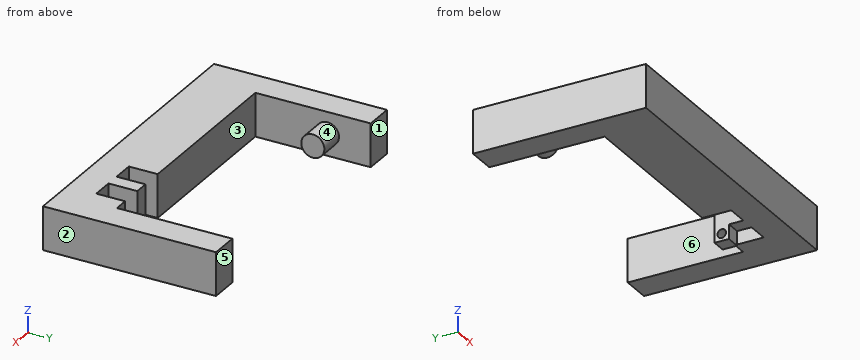
```python
from build123d import *

# Parameters (mm, degrees)
SKETCH1_3_W           = 7.5
SKETCH1_3_H           = 15
BOSS_EXTRUDE2_DEPTH   = 10
BOSS_EXTRUDE2_2_DEPTH = 10
SKETCH1_W             = 5
SKETCH1_H             = 15
SKETCH1_W_2           = 60
BOSS_EXTRUDE3_DEPTH   = 20
SKETCH2_W             = 5
SKETCH2_H             = 5
BOSS_EXTRUDE5_DEPTH   = 5
SKETCH1_9_W           = 10
SKETCH1_9_H           = 15
BOSS_EXTRUDE6_DEPTH   = 60
SKETCH4_R             = 4
BOSS_EXTRUDE7_DEPTH   = 9
SKETCH5_R             = 1.5
CUT_EXTRUDE1_DEPTH    = 5


with BuildPart() as part:
    # Sketch1<3> → Boss-Extrude2 (new body)
    with BuildSketch(Plane(origin=(0, 0, 0), x_dir=(1, 0, 0), z_dir=(0, 1, 0))):
        with Locations((36.25, 0)):
            Rectangle(SKETCH1_3_W, SKETCH1_3_H)
    extrude(amount=BOSS_EXTRUDE2_DEPTH)



with BuildPart() as body_2:
    # Sketch1<3> → Boss-Extrude2 2 (new body)
    with BuildSketch(Plane(origin=(0, 0, 0), x_dir=(1, 0, 0), z_dir=(0, 1, 0))):
        with Locations((23.75, 0)):
            Rectangle(SKETCH1_3_W, SKETCH1_3_H)
    extrude(amount=BOSS_EXTRUDE2_2_DEPTH)


with BuildPart() as part_1:
    add(part.part)

    add(body_2.part)  # Boss-Extrude3 merges body 2
    # Sketch1 → Boss-Extrude3 (add)
    with BuildSketch(Plane(origin=(0, 0, 0), x_dir=(1, 0, 0), z_dir=(0, 1, 0))):
        with Locations((30, 0)):
            Rectangle(SKETCH1_W, SKETCH1_H)
        with Locations((-10, 0)):
            Rectangle(SKETCH1_W_2, SKETCH1_H)
        with Locations((42.5, 0)):
            Rectangle(SKETCH1_W, SKETCH1_H)
    extrude(amount=BOSS_EXTRUDE3_DEPTH)

    # Sketch2 → Boss-Extrude5 (add)
    with BuildSketch(Plane(origin=(0, 0, -7.5), x_dir=(-1, 0, 0), z_dir=(0, 0, -1))):
        with Locations((-30, 17.5)):
            Rectangle(SKETCH2_W, SKETCH2_H)
    extrude(amount=BOSS_EXTRUDE5_DEPTH)

    # Sketch1<9> → Boss-Extrude6 (add)
    with BuildSketch(Plane(origin=(0, 0, 0), x_dir=(1, 0, 0), z_dir=(0, 1, 0))):
        with Locations((50, 0)):
            Rectangle(SKETCH1_9_W, SKETCH1_9_H)
        with Locations((-45, 0)):
            Rectangle(SKETCH1_9_W, SKETCH1_9_H)
    extrude(amount=BOSS_EXTRUDE6_DEPTH)

    # Sketch4 → Boss-Extrude7 (add)
    with BuildSketch(Plane(origin=(-40, 0, 0), x_dir=(0, 0, -1), z_dir=(1, 0, 0))):
        with Locations((0, 45)):
            Circle(SKETCH4_R)
    extrude(amount=BOSS_EXTRUDE7_DEPTH)

    # Sketch5 → Cut-Extrude1 (cut)
    with BuildSketch(Plane(origin=(32.5, 0, 0), x_dir=(0, 0, -1), z_dir=(1, 0, 0))):
        with Locations((10, 17.5)):
            Circle(SKETCH5_R)
    extrude(amount=-CUT_EXTRUDE1_DEPTH, mode=Mode.SUBTRACT)


solid = part_1.part
```
The model under review builds one solid part; all positions refer to its coordinate system, in mm. Face numbers are marked on the shaded views. A direction names the side the tool comes from. Round coordinates to 2 decimals unless told otherwise and drop trailing zeros. Loops run counter-clockwise (first coordinate to the right, second up) from the corner with the lowest first, then second, coordinate; pieces in that order, holes last. Notation, with made-up numbers: (28, 44) -> (52, 44) arc R8 ccw to (52, 55) -> close; hole circle Ø9 at (35, 84). An arc over 180 degrees is marked (long way). Answer as a JSON object with one key per item and string values. Group by question number.
1) We need section D-D on z = 0. Write out the cut boundary in (x, y), then the cut area to 3 significant figures.
2) For line 1 (X direction, y = 17, z = -4); line 2 (X direction, y = 37.5, z = 1.25); line 3 (Y direction, x = 30.7, z = -10), list the stretches that pass through material, from the lowest coordinate up. Write a range as [from, to].
3) We need section B-B on y = 45. Write out the cut boundary in (x, z), then the cut area to 3 significant figures.
4) For the marked faces 4, 5 and 6, list the 3-axis set-ups (+Z, -Z, +X, -X, +Y, -Y) from which the entire face can be reached by the end or side of a thin tool; tool diameter is ignored.
5) For pin 1 Ø1.5 at (x, z) = (11.5, -7) entering from +Y; pin 2 Ø18 at (x, y) = (17, 18) entering from -Z; pin 3 Ø4 at (x, z) = (23, 1) entering from +Y, all flat-tipped, find the tip position at first contact; note any pin that passes through.
6) Mouldability with a two-part tool opening along X and no side actions: class the marked faces 1, 2 and 3 as released by +X, released by -X, zero draft, split by the parting line, or undercut.
7) We need section A-A on y = 17.5. Write out the cut boundary in (x, z).
8) We need section C-C on z = -10. Write out the cut boundary in (x, y).
Result set:
{
 "1": {"outline": "(-50, 0) -> (55, 0) -> (55, 60) -> (45, 60) -> (45, 20) -> (40, 20) -> (40, 10) -> (32.5, 10) -> (32.5, 20) -> (27.5, 20) -> (27.5, 10) -> (20, 10) -> (20, 20) -> (-40, 20) -> (-40, 41) -> (-31, 41) -> (-31, 49) -> (-40, 49) -> (-40, 60) -> (-50, 60) -> close", "area": "2,820 mm²"},
 "2": {"line 1": "[-50, 20], [27.5, 32.5], [40, 55]", "line 2": "[-50, -40], [45, 55]", "line 3": "[15, 16], [19, 20]"},
 "3": {"outline": "(-50, -7.5) -> (-40, -7.5) -> (-40, -4) -> (-31, -4) -> (-31, 4) -> (-40, 4) -> (-40, 7.5) -> (-50, 7.5) -> close; (45, -7.5) -> (55, -7.5) -> (55, 7.5) -> (45, 7.5) -> close", "area": "372 mm²"},
 "4": {"face 4": "none", "face 5": "+Z, -Z, +X, -X, +Y", "face 6": "+Z, -Z, +Y"},
 "5": {"pin 1": "y = 20", "pin 2": "z = -7.5", "pin 3": "y = 10"},
 "6": {"face 1": "zero draft", "face 2": "released by +X", "face 3": "undercut"},
 "7": {"outline": "(-50, -7.5) -> (20, -7.5) -> (20, 7.5) -> (-50, 7.5) -> close; (27.5, -12.5) -> (32.5, -12.5) -> (32.5, -11.5) -> (27.5, -11.5) -> close; (27.5, -8.5) -> (32.5, -8.5) -> (32.5, 7.5) -> (27.5, 7.5) -> close; (40, -7.5) -> (55, -7.5) -> (55, 7.5) -> (40, 7.5) -> close"},
 "8": {"outline": "(27.5, 15) -> (32.5, 15) -> (32.5, 16) -> (27.5, 16) -> close; (27.5, 19) -> (32.5, 19) -> (32.5, 20) -> (27.5, 20) -> close"}
}
